from build123d import *

# Parameters (mm, degrees)
SKETCH1_W           = 6
SKETCH1_H           = 6
BOSS_EXTRUDE1_DEPTH = 19
SKETCH2_R           = 1.8
CUT_EXTRUDE1_DEPTH  = 5
FILLET1_R           = 1


with BuildPart() as part:
    # Sketch1 → Boss-Extrude1 (new body)
    with BuildSketch(Plane.XY):
        Rectangle(SKETCH1_W, SKETCH1_H)
    extrude(amount=BOSS_EXTRUDE1_DEPTH)

    # Sketch2 → Cut-Extrude1 (cut)
    with BuildSketch(Plane(origin=(0, 0, 0), x_dir=(-1, 0, 0), z_dir=(0, 0, -1))):
        Circle(SKETCH2_R)
    extrude(amount=-CUT_EXTRUDE1_DEPTH, mode=Mode.SUBTRACT)

    # Fillet1
    fillet1_edges = [part.edges().sort_by_distance(p)[0] for p in [
        (3, 0, 19),
        (0, 3, 19),
        (-3, 0, 19),
        (0, -3, 19),
    ]]
    fillet(fillet1_edges, radius=FILLET1_R)


solid = part.part
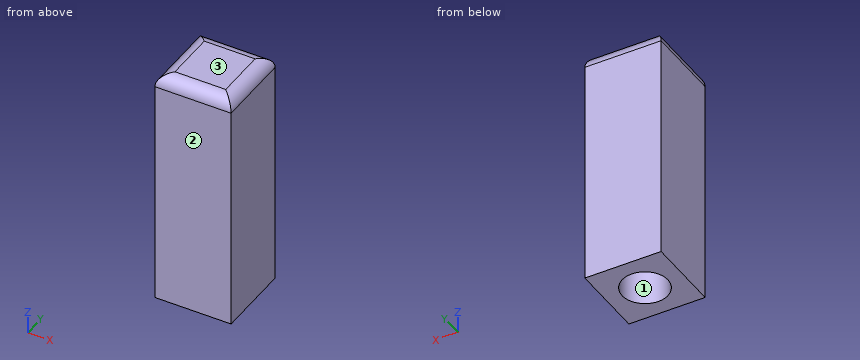
For this review, take the finished solid that the model builds, in its own axes (mm). Face numbers are marked on the shaded views. Round coordinates to 2 decimals unless told otherwise and drop trailing zeros. Write each loop counter-clockwise with the first axis right and the second up, starting at its lowest first coordinate (ties: lowest second). Pieces come first, ordered by that corner, then holes. Notation, with made-up numbers: (-21.75, 47.25) - (-3.75, 47.25) arc R14 ccw to (-3.75, 68.25) - close; hole circle Ø1 at (65, 51). An arc over 180 degrees is marked (long way). Write item = value, one per line. Start each with the question number.
1. Consider section B-B on z = 2.25. State the section outline as (x, y) points, plus the area to 3 significant figures.
2. For pin 1 Ø1.8 at (x, y) = (0.5, -0.5) entering from -Z, flat-tipped, find the tip position at first contact; note if it passes through.
3. Consider section A-A on x = 0. State the section outline as (y, z) points.
4. Wall thickness on L1, parallel to Y at x = 0, z = 3.15; L2, parallel to Y at x = -0.95, z = 4.25; L3, parallel to Z at x = 0.3, y = -1.1: over which ranges is each line inside the solid? List them lowest first.
5. Draft analysis for pull direction Y (two halves, no side actions). For the marked faces 1, 2 and 3, state which applies: released by +Y, released by -Y, zero draft, split by the parting line, or undercut.
Evaluation:
q1.outline = (-3, -3) - (3, -3) - (3, 3) - (-3, 3) - close; hole circle Ø3.6 at (0, 0)
q1.area = 25.8 mm2
q2.pin_1 = 5
q3.outline = (-3, 0) - (-1.8, 0) - (-1.8, 5) - (1.8, 5) - (1.8, 0) - (3, 0) - (3, 18) arc R1 ccw to (2, 19) - (-2, 19) arc R1 ccw to (-3, 18) - close
q4.L1 = -3 to -1.8, 1.8 to 3
q4.L2 = -3 to -1.53, 1.53 to 3
q4.L3 = 5 to 19
q5.face_1 = undercut
q5.face_2 = released by -Y
q5.face_3 = zero draft
